from build123d import *

# Parameters (mm, degrees)
BOSS_EXTRUDE1_DEPTH = 5
CUT_EXTRUDE1_REACH  = 91.582
CUT_EXTRUDE2_REACH  = 91.582
SKETCH3_R           = 2.525
FILLET1_R           = 3
FILLET2_R           = 3


with BuildPart() as part:
    # Sketch1 → Boss-Extrude1 (new body)
    with BuildSketch(Plane.XY):
        Polygon((20, 40), (80, 40), (80, 0), (20, 0), (0, 0), (0, 20), (0, 40), align=None)
    extrude(amount=BOSS_EXTRUDE1_DEPTH)

    # Sketch2 → Cut-Extrude1 (cut, up to next)
    with BuildSketch(Plane.XY.offset(5), mode=Mode.PRIVATE) as cut_extrude1_sk1:
        Polygon((20, 15.958548116), (23.5, 17.979274058), (23.5, 22.020725942), (20, 24.041451884), (16.5, 22.020725942), (16.5, 17.979274058), align=None)
    cut_extrude1_tool1 = extrude(cut_extrude1_sk1.sketch, amount=-CUT_EXTRUDE1_REACH, mode=Mode.PRIVATE) & part.part
    add(cut_extrude1_tool1.solids().sort_by_distance((20, 20, 5))[0], mode=Mode.SUBTRACT)

    # Sketch3 → Cut-Extrude2 (cut, up to next)
    with BuildSketch(Plane.XY.offset(5), mode=Mode.PRIVATE) as cut_extrude2_sk1:
        with Locations((55, 30)):
            Circle(SKETCH3_R)
    cut_extrude2_tool1 = extrude(cut_extrude2_sk1.sketch, amount=-CUT_EXTRUDE2_REACH, mode=Mode.PRIVATE) & part.part
    # Sketch3 → Cut-Extrude2 (cut, up to next)
    with BuildSketch(Plane.XY.offset(5), mode=Mode.PRIVATE) as cut_extrude2_sk2:
        with Locations((55, 10)):
            Circle(SKETCH3_R)
    cut_extrude2_tool2 = extrude(cut_extrude2_sk2.sketch, amount=-CUT_EXTRUDE2_REACH, mode=Mode.PRIVATE) & part.part
    # Sketch3 → Cut-Extrude2 (cut, up to next)
    with BuildSketch(Plane.XY.offset(5), mode=Mode.PRIVATE) as cut_extrude2_sk3:
        with Locations((70, 30)):
            Circle(SKETCH3_R)
    cut_extrude2_tool3 = extrude(cut_extrude2_sk3.sketch, amount=-CUT_EXTRUDE2_REACH, mode=Mode.PRIVATE) & part.part
    # Sketch3 → Cut-Extrude2 (cut, up to next)
    with BuildSketch(Plane.XY.offset(5), mode=Mode.PRIVATE) as cut_extrude2_sk4:
        with Locations((70, 10)):
            Circle(SKETCH3_R)
    cut_extrude2_tool4 = extrude(cut_extrude2_sk4.sketch, amount=-CUT_EXTRUDE2_REACH, mode=Mode.PRIVATE) & part.part
    add(cut_extrude2_tool1.solids().sort_by_distance((55, 30, 5))[0], mode=Mode.SUBTRACT)
    add(cut_extrude2_tool2.solids().sort_by_distance((55, 10, 5))[0], mode=Mode.SUBTRACT)
    add(cut_extrude2_tool3.solids().sort_by_distance((70, 30, 5))[0], mode=Mode.SUBTRACT)
    add(cut_extrude2_tool4.solids().sort_by_distance((70, 10, 5))[0], mode=Mode.SUBTRACT)

    # Fillet1
    fillet1_edges = [part.edges().sort_by_distance(p)[0] for p in [
        (80, 40, 2.5),
        (80, 0, 2.5),
    ]]
    fillet(fillet1_edges, radius=FILLET1_R)

    # Fillet2
    fillet2_edges = [part.edges().sort_by_distance(p)[0] for p in [
        (0, 0, 2.5),
        (0, 40, 2.5),
    ]]
    fillet(fillet2_edges, radius=FILLET2_R)


solid = part.part
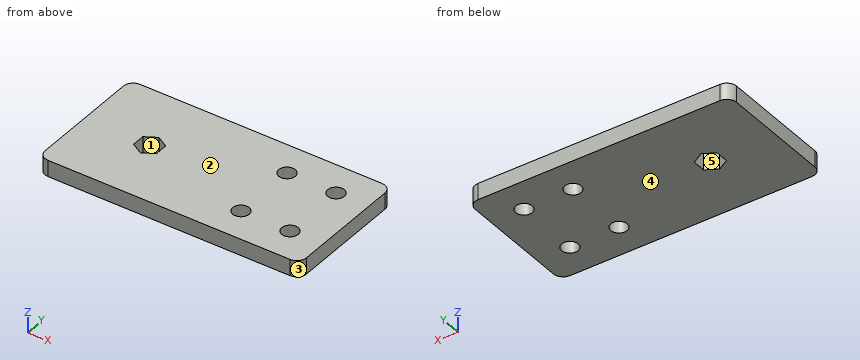
Geometry: final body of the model. Coordinates: model frame, mm. Face numbers are marked on the shaded views. A direction names the side the tool comes from. Give positions to 0.01 mm unless a question says otherwise; leave off trailing zeros. Loops run counter-clockwise (first coordinate to the right, second up) from the corner with the lowest first, then second, coordinate; pieces in that order, holes last. Notation, with made-up numbers: (-15.5, 48) - (28.5, 48) arc R10 cw to (28.5, 65) - close; hole circle Ø2 at (30.25, -23). An arc over 180 degrees is marked (long way). One line per question, with ' | ' between items. Start each with the question number.
(1) Section query B-B on y = 10. Return loops of the section in (x, z) (3 decimals).
(2) Section query A-A on x = 70. Return loops of the section in (y, z) (3 decimals).
(3) Section query C-C on z = 3.4. Return loops of the section in (x, y) (3 decimals), then the cut area to 3 significant figures.
(4) Ray query, line 1 (Y direction, x = 55, z = 2.8) (3 decimals); line 2 (X direction, y = 21.5, z = 2.2); line 3 (Y direction, x = 68.5, z = 1.7). Return the intervals inside material, ascending. Write a range as from..to.
(5) Reachability of the marked faces 4 and 5 from +Z, -Z, +X, -X, +Y, -Y: full face, straight path, thin tool, end or side. Return the list, or none.
(6) Pull-direction query (X, two-part tool) for the marked faces 1, 2 and 3; classes: released by +X, released by -X, zero draft, split by the parting line, or undercut.
The answers:
1) outline: (0, 0) - (52.475, 0) - (52.475, 5) - (0, 5) - close; (57.525, 0) - (67.475, 0) - (67.475, 5) - (57.525, 5) - close; (72.525, 0) - (80, 0) - (80, 5) - (72.525, 5) - close
2) outline: (0, 0) - (7.475, 0) - (7.475, 5) - (0, 5) - close; (12.525, 0) - (27.475, 0) - (27.475, 5) - (12.525, 5) - close; (32.525, 0) - (40, 0) - (40, 5) - (32.525, 5) - close
3) outline: (0, 3) arc R3 ccw to (3, 0) - (77, 0) arc R3 ccw to (80, 3) - (80, 37) arc R3 ccw to (77, 40) - (3, 40) arc R3 ccw to (0, 37) - close; hole (16.5, 17.979) - (20, 15.959) - (23.5, 17.979) - (23.5, 22.021) - (20, 24.041) - (16.5, 22.021) - close; hole circle Ø5.05 at (55, 10); hole circle Ø5.05 at (55, 30); hole circle Ø5.05 at (70, 10); hole circle Ø5.05 at (70, 30) | area: 3,070 mm2
4) line 1: 0..7.475, 12.525..27.475, 32.525..40 | line 2: 0..16.5, 23.5..80 | line 3: 0..7.97, 12.03..27.97, 32.03..40
5) face 4: -Z, +X, -X, +Y, -Y | face 5: +Z, -Z
6) face 1: undercut | face 2: zero draft | face 3: released by +X
